```python
from build123d import *

# Parameters (mm, degrees)
BOSS_EXTRUDE1_DEPTH = 0.41
BOSS_EXTRUDE2_DEPTH = 0.4
BOSS_EXTRUDE3_DEPTH = 10


with BuildPart() as part:
    # Sketch1 → Boss-Extrude1 (new body)
    with BuildSketch(Plane.XY):
        Polygon((-5.5, 17), (-5.5, 71.298294078), (-39.578838325, 90.973720558), (-34.078838325, 100.5), (-5.5, 84), (-5.5, 117), (5.5, 117), (5.5, 84), (34.078838325, 100.5), (39.578838325, 90.973720558), (5.5, 71.298294078), (5.5, 17), (6.3, 17), (6.3, 70.836413862), (40.671658648, 90.680900235), (34.371658648, 101.592820323), (6.3, 85.385640646), (6.3, 117.8), (-6.3, 117.8), (-6.3, 85.385640646), (-34.371658648, 101.592820323), (-40.671658648, 90.680900235), (-6.3, 70.836413862), (-6.3, 17), align=None)
    extrude(amount=BOSS_EXTRUDE1_DEPTH)

    # Sketch2 → Boss-Extrude2 (add)
    with BuildSketch(Plane.XY):
        Polygon((-5.5, 17), (-5.5, 71.298294078), (-39.578838325, 90.973720558), (-34.078838325, 100.5), (-5.5, 84), (-5.5, 117), (5.5, 117), (5.5, 84), (34.078838325, 100.5), (39.578838325, 90.973720558), (5.5, 71.298294078), (5.5, 17), align=None)
    extrude(amount=BOSS_EXTRUDE2_DEPTH)

    # Sketch3 → Boss-Extrude3 (add)
    with BuildSketch(Plane.XY):
        Polygon((-6.3, 17.2), (-6.3, 70.836413862), (-40.671658648, 90.680900235), (-34.371658648, 101.592820323), (-6.3, 85.385640646), (-6.3, 117.8), (6.3, 117.8), (6.3, 85.385640646), (34.371658648, 101.592820323), (40.671658648, 90.680900235), (6.3, 70.836413862), (6.3, 17.2), (7.1, 17.2), (7.1, 70.374533647), (41.764478971, 90.388079912), (34.664478971, 102.685640646), (7.1, 86.771281292), (7.1, 118.6), (-7.1, 118.6), (-7.1, 86.771281292), (-34.664478971, 102.685640646), (-41.764478971, 90.388079912), (-7.1, 70.374533647), (-7.1, 17.2), align=None)
    extrude(amount=BOSS_EXTRUDE3_DEPTH)


solid = part.part
```
Read the model definition and answer for the solid it produces. Units are mm, in the model's axes. A direction names the side the tool comes from. Give positions to 0.01 mm unless a question says otherwise; leave off trailing zeros. Write each loop counter-clockwise with the first axis right and the second up, starting at its lowest first coordinate (ties: lowest second). Pieces come first, ordered by that corner, then holes. Notation, with made-up numbers: M -34.75,-11 L -21.75,-11 A8 ccw -21.75,1 Z; hole C 21,75.5 d5. An arc over 180 degrees is marked long. Put each result on its own line as item: value. Start each with the question number.
1. The part is cut by section C-C, the plane z = 6.75. Give the vertices of the cut face in (x, y).
2. Which of the six approach directions +Z, -Z, +X, -X, +Y, -Y give full straight-line access (tool end or side, diameter ignored) to faces 4 (the flat face through (3, 76, 0)), 5 (the flat face through (-23.245, 80.62, 5.138)), 6 (the flat face through (24.19, 80.24, 4.93)), 7 (the flat face through (21.075, 94.84, 4.93)), 8 (the flat face through (-6.3, 44, 5))?
3. For a pull along Y with two mould halves and no side action, classify faces 1 (the flat face through (0, 78, 0.4)), 2 (the flat face through (-38.165, 96.623, 4.93)), 3 (the flat face through (-7.1, 103, 5)) as released by +Y, released by -Y, zero draft, split by the parting line, or undercut.
4. Each of these flat-tipped pins is pushed along its axis until it touches: pin 1 Ø2 at (y, z) = (49, 5.5) entering from +X; pin 2 Ø0.9 at (x, z) = (6.5, 6) entering from -Y; pin 3 Ø3 at (x, z) = (2, 7) entering from -Y. Where does it stop, or does it pass through?
5. Consider line 1 along X through (y, z) = (41.5, 5); line 2 along X through (y, z) = (89, 3.5); line 3 along X through (y, z) = (93.5, 1.75). Determine where each line is inside the solid, lowest interval first.
Final values:
1. outline: M -41.76,90.39 L -7.1,70.37 L -7.1,17.2 L -6.3,17.2 L -6.3,70.84 L -40.67,90.68 L -34.37,101.59 L -6.3,85.39 L -6.3,117.8 L 6.3,117.8 L 6.3,85.39 L 34.37,101.59 L 40.67,90.68 L 6.3,70.84 L 6.3,17.2 L 7.1,17.2 L 7.1,70.37 L 41.76,90.39 L 34.66,102.69 L 7.1,86.77 L 7.1,118.6 L -7.1,118.6 L -7.1,86.77 L -34.66,102.69 Z
2. face 4: -Z, +X, -X, +Y, -Y
2. face 5: +Z
2. face 6: +Z, -Z, +X, -Y
2. face 7: +Z, -Z, +Y
2. face 8: +Z, -Y
3. face 1: undercut
3. face 2: released by +Y
3. face 3: zero draft
4. pin 1: stops at x = 7.1
4. pin 2: stops at y = 17.2
4. pin 3: stops at y = 117.8
5. line 1: x = -7.1 to -6.3, 6.3 to 7.1
5. line 2: x = -39.36 to -37.76, -12.56 to -10.96, -7.1 to -6.3, 6.3 to 7.1, 10.96 to 12.56, 37.76 to 39.36
5. line 3: x = -39.97 to -39.04, -20.35 to -18.75, -7.1 to -6.3, 6.3 to 7.1, 18.75 to 20.35, 39.04 to 39.97
